Can you work these out from the model? Positions are in its coordinate system, mm. A direction names the side the tool comes from. Round coordinates to 2 decimals unless told otherwise and drop trailing zeros. Loops run counter-clockwise (first coordinate to the right, second up) from the corner with the lowest first, then second, coordinate; pieces in that order, holes last. Notation, with made-up numbers: M -8.75,43 L 21.25,43 A14 cw 21.25,53 Z; hole C 32,88.5 d4. An arc over 180 degrees is marked long. Answer as CSV lines item,"result".
from build123d import *

# Parameters (mm, degrees)
SKETCH1_R           = 31.75
BOSS_EXTRUDE1_DEPTH = 19.05
SKETCH2_R           = 2.9845
CUT_EXTRUDE1_DEPTH  = 12.7
CHAMFER1_SIZE       = 1.905


with BuildPart() as part:
    # Sketch1 → Boss-Extrude1 (new body)
    with BuildSketch(Plane(origin=(0, 0, 0), x_dir=(0, 0, -1), z_dir=(1, 0, 0))):
        with Locations(Location((0, 0, 0), (0, 0, 180))):
            Circle(SKETCH1_R)
    extrude(amount=BOSS_EXTRUDE1_DEPTH)

    # Sketch2 → Cut-Extrude1 (cut)
    with BuildSketch(Plane.ZY):
        Circle(SKETCH2_R)
    extrude(amount=-CUT_EXTRUDE1_DEPTH, mode=Mode.SUBTRACT)

    # Chamfer1
    chamfer1_edges = [part.edges().sort_by_distance(p)[0] for p in [
        (0, 0, -31.75),
        (19.05, 0, -31.75),
    ]]
    chamfer(chamfer1_edges, length=CHAMFER1_SIZE)


solid = part.part
Item 1: We'd pull the mould along Z, two halves only. Please class faces 3 (the face through (0, 6, 0)), 4 (the face through (12.7, 0, 0)), 5 (the face through (9.418, 30.995, -6.883)): released by +Z, released by -Z, zero draft, split by the parting line, or undercut.
Output:
face 3,"zero draft"
face 4,"undercut"
face 5,"split by the parting line"
Item 2: If I drill on line 1 along Y through (x, z) = (9, 0); line 2 along Z through (x, y) = (9.25, 23); line 3 along X through (y, z) = (-29, -11), over which ranges is the centre line in solid material (lowest first)? Write a range as from..to.
Output:
line 1,"y = -31.75..-2.98, 2.98..31.75"
line 2,"z = -21.89..21.89"
line 3,"x = 1.17..17.88"
Item 3: If we section it at C-C on x = 7.25: Write out the boundary of the cut face in (y, z), then the cut area to 3 significant figures.
Output:
outline,"C 0,0 d63.5; hole C 0,0 d5.97"
area,"3,140 mm2"
Item 4: Will these pins go through, and if not, where does the flat tip stop? pin 1 (5 mm diameter, centred on x = 10.5, z = 5.5, fed in from -Y); pin 2 (5 mm diameter, centred on x = 11.5, y = 20.5, fed in from +Z); pin 3 (5 mm diameter, centred on x = 10.5, y = -19.5, fed in from +Z).
Output:
pin 1,"stops at y = -31.61"
pin 2,"stops at z = 26.15"
pin 3,"stops at z = 26.82"
Item 5: On a 3-axis mill with a long thin cutter (end or side, diameter ignored), from which of +Z, -Z, +X, -X, +Y, -Y can I reach the whole of each face in a straight line? I mean faces 1 (the face through (19.05, 0, 0)), 2 (the face through (6.261, -2.914, -0.647)). Say none if no direction works.
Output:
face 1,"+Z, -Z, +X, +Y, -Y"
face 2,"-X"
